Autodesk Fusion 360 part; units mm, degrees
sketch "Sketch3" plane through (0, 0, 0) normal (0, 1, 0) x (1, 0, 0)
  line L0 (42, -10) -> (120, -10)
  line L1 (135, -25) -> (135, -59)
  line L2 (120, -74) -> (42, -74)
  line L3 (10, -42) -> (10, -42)
  arc A0 (42, -10) -> (10, -42) centre (42, -42) ccw
  arc A1 (10, -42) -> (42, -74) centre (42, -42) ccw
  arc A2 (135, -25) -> (120, -10) centre (120, -25) ccw
  arc A3 (120, -74) -> (135, -59) centre (120, -59) ccw
  circle A4 centre (120, -59) radius 6.5
  circle A5 centre (120, -25) radius 6.5
  point P0 (10, -10)
  point P1 (135, -10)
  point P2 (10, -74)
  dimension "d17" = 125
  dimension "d18" = 64
  dimension "d19" = 32
  dimension "d20" = 32
  dimension "d21" = 15
  dimension "d22" = 15
  dimension "d23" = 13
  dimension "d24" = 13
extrude "Extrude3" add sketch "Sketch3" along normal blind 20
sketch "Sketch4" plane through (0, 20, 0) normal (0, 1, 0) x (-1, 0, 0)
  circle A0 centre (-120, 59) radius 6.5
  circle A1 centre (-120, 25) radius 6.5
  arc A2 (-42, 10) -> (-42, 74) centre (-42, 42) ccw
  line L0 (-42, 74) -> (-120, 74)
  arc A3 (-120, 74) -> (-135, 59) centre (-120, 59) ccw
  line L1 (-135, 59) -> (-135, 25)
  arc A4 (-135, 25) -> (-120, 10) centre (-120, 25) ccw
  line L2 (-120, 10) -> (-42, 10)
  line L3 (-120, 59) -> (-72, 59)
  line L4 (-120, 25) -> (-72, 25)
  line L5 (-72, 59) -> (-72, 25)
  line L6 (-72, 59) -> (-72, 42)
  circle A5 centre (-72, 42) radius 30
  dimension "d27" = 48
  dimension "d28" = 48
  dimension "d29" = 60
extrude "Extrude4" add sketch "Sketch4" along normal blind 45 contours L3 L4 L5 L6 A5 | L3 L4 L5 L6 A5
hole "Hole1" at (72, 65, 42) direction (0, -1, 0) diameter 30 depth 90 tip angle 118
sketch "Sketch5" plane through (0, 0, 74) normal (0, 0, 1) x (1, 0, 0)
  line L0 (42, 0) -> (120, 0)
  line L1 (120, 0) -> (120, 20)
  line L2 (120, 20) -> (42, 20)
  line L3 (42, 20) -> (42, 0)
sketch "Sketch6" plane through (0, 0, 0) normal (0, 0, 1) x (1, 0, 0)
  line L0 (42, 65) -> (72, 65)
  line L1 (42, 65) -> (42, 57.5)
  line L2 (42, 57.5) -> (57, 57.5)
  line L3 (57, 57.5) -> (87, 57.5)
  line L4 (87, 57.5) -> (87, 27.5)
  line L5 (87, 27.5) -> (57, 27.5)
  line L6 (57, 27.5) -> (57, 57.5)
  dimension "d35" = 30
  dimension "d36" = 7.5
  dimension "d37" = 30
  dimension "d38" = 30
extrude "Extrude5" cut sketch "Sketch6" along normal blind 200
sketch "Sketch7" plane through (0, 0, 0) normal (0, 1, 0) x (1, 0, 0)
sketch "Sketch8" plane through (0, 20, 0) normal (0, 1, 0) x (-1, 0, 0)
  circle A0 centre (-72, 42) radius 30
  circle A1 centre (-120, 59) radius 6.5
  circle A2 centre (-120, 25) radius 6.5
  arc A3 (-42, 10) -> (-42, 74) centre (-42, 42) ccw
  line L0 (-42, 74) -> (-120, 74)
  arc A4 (-120, 74) -> (-135, 59) centre (-120, 59) ccw
  line L1 (-135, 59) -> (-135, 25)
  arc A5 (-135, 25) -> (-120, 10) centre (-120, 25) ccw
  line L2 (-120, 10) -> (-42, 10)
  line L3 (-72, 42) -> (-27, 42)
  circle A6 centre (-27, 42) radius 6.5
  dimension "d41" = 45
  dimension "d42" = 13
extrude "Extrude6" cut sketch "Sketch8" against normal blind 9 contours A6
sketch "Sketch9" plane through (0, 20, 0) normal (0, 1, 0) x (-1, 0, 0)
  circle A0 centre (-27, 42) radius 6.5
  circle A1 centre (-72, 42) radius 30
  circle A2 centre (-120, 59) radius 6.5
  circle A3 centre (-120, 25) radius 6.5
  arc A4 (-42, 10) -> (-42, 74) centre (-42, 42) ccw
  line L0 (-42, 74) -> (-120, 74)
  arc A5 (-120, 74) -> (-135, 59) centre (-120, 59) ccw
  line L1 (-135, 59) -> (-135, 25)
  arc A6 (-135, 25) -> (-120, 10) centre (-120, 25) ccw
  line L2 (-120, 10) -> (-42, 10)
  line L3 (-27, 42) -> (-27, 31)
  line L4 (-27, 31) -> (-6.9654, 31)
  line L5 (-6.9654, 31) -> (-6.9654, 50)
  line L6 (-6.9654, 50) -> (-6.9654, 31)
  line L7 (-27, 42) -> (-27, 53)
  line L8 (-27, 53) -> (-28, 53)
  line L9 (-38, 43) -> (-38, 41)
  line L10 (-38, 31) -> (-27, 31)
  line L11 (-27, 31) -> (-27, 53)
  line L12 (-28, 31) -> (-6, 31)
  line L13 (-6, 31) -> (-6, 53)
  line L14 (-6, 53) -> (-38, 53)
  line L15 (-38, 53) -> (-38, 31)
  arc A7 (-38, 41) -> (-28, 31) centre (-28, 41) ccw
  arc A8 (-28, 53) -> (-38, 43) centre (-28, 43) ccw
  point P0 (-38, 53)
  dimension "d45" = 11
  dimension "d46" = 11
  dimension "d47" = 11
  dimension "d48" = 22
  dimension "d49" = 32
  dimension "d50" = 22
  dimension "d51" = 10
  dimension "d52" = 10
extrude "Extrude7" cut sketch "Sketch9" against normal blind 9 contours A0 A4 L3 L4 L7 L11 L12 L14 | A0 L3 L7 L8 L9 L10 L11 L12 L14 L15 A7 A8
hole "Hole2" at (27.171, 11, 42.0282) direction (0, -1, 0) diameter 12 depth 13 tip angle 118
Read the model definition and answer for the solid it produces. Units are mm, in the model's axes. A direction names the side the tool comes from. Round coordinates to 2 decimals unless told otherwise and drop trailing zeros. Loops run counter-clockwise (first coordinate to the right, second up) from the corner with the lowest first, then second, coordinate; pieces in that order, holes last. Notation, with made-up numbers: (61.5, 86.5) -> (68.5, 86.5) arc R30 cw to (68.5, 120.5) -> close; hole circle Ø6 at (40.5, 58). An arc over 180 degrees is marked (long way). One line per item, written item: value.
1) A cutting plane is placed at C-C (z = 46). Determine the outline of the cut face in (x, y).
Answer list:
outline: (10.25, 0) -> (22.67, 0) -> (22.67, 11) -> (10.25, 11) -> close; (31.67, 0) -> (57.54, 0) -> (57.54, 27.5) -> (57, 27.5) -> (57, 57.5) -> (57.54, 57.5) -> (57.54, 65) -> (42.27, 65) -> (42.27, 20) -> (37.54, 20) -> (37.54, 11) -> (31.67, 11) -> close; (86.46, 0) -> (135, 0) -> (135, 20) -> (101.73, 20) -> (101.73, 65) -> (86.46, 65) -> (86.46, 57.5) -> (87, 57.5) -> (87, 27.5) -> (86.46, 27.5) -> close
2) A cutting plane is placed at D-D (y = 9). Determine the outline of the cut face in (x, z).
Answer list:
outline: (42, 10) -> (120, 10) arc R15 ccw to (135, 25) -> (135, 59) arc R15 ccw to (120, 74) -> (42, 74) arc R32 ccw to start; hole circle Ø12 at (27.17, 42.03); hole circle Ø30 at (72, 42); hole circle Ø13 at (120, 25); hole circle Ø13 at (120, 59)
3) A cutting plane is placed at B-B (z = 64). Determine the outline of the cut face in (x, y).
Answer list:
outline: (18.76, 0) -> (115.85, 0) -> (115.85, 20) -> (92.4, 20) -> (92.4, 65) -> (51.6, 65) -> (51.6, 20) -> (18.76, 20) -> close; (124.15, 0) -> (134.14, 0) -> (134.14, 20) -> (124.15, 20) -> close; hole (57, 27.5) -> (87, 27.5) -> (87, 57.5) -> (57, 57.5) -> close
4) The mould has two halves that part along Y. Classify faces 4 (the face through (72, 57.5, 63)), 5 (the face through (100, 20, 56)), 6 (the face through (34.99, 15.56, 50.15)): pulls with the +Y half, pulls with the -Y half, needs draft (parallel to the pull), parting line crosses it, or undercut.
Answer list:
face 4: undercut
face 5: pulls with the +Y half
face 6: needs draft
5) For faces 1 (the face through (114.842, 9.86, 55.045)), 2 (the face through (20, 16, 31)), 3 (the face through (87, 43, 42)), determine the directions among +Z, -Z, +X, -X, +Y, -Y from which every point of the face is accessible in a straight line to the end or side of a thin tool.
Answer list:
face 1: +Y, -Y
face 2: -X, +Y
face 3: +Z, -Z
6) Consider L1, parallel to Z at x = 120, y = 5; L2, parallel to X at y = 60, z = 42; L3, parallel to Z at x = 72, y = 61.25. Determine where each line is inside the solid, lowest interval first. Write a range as [from, to].
Answer list:
L1: z = [10, 18.5], [31.5, 52.5], [65.5, 74]
L2: x = [42, 57], [87, 102]
L3: z = [12, 27], [57, 72]
7) A cutting plane is placed at A-A (x = 72). Determine the outline of the cut face in (y, z), and give its area (3 significant figures).
Answer list:
outline: (0, 10) -> (20, 10) -> (20, 12) -> (27.5, 12) -> (27.5, 27) -> (0, 27) -> close; (0, 57) -> (27.5, 57) -> (27.5, 72) -> (20, 72) -> (20, 74) -> (0, 74) -> close; (57.5, 12) -> (65, 12) -> (65, 27) -> (57.5, 27) -> close; (57.5, 57) -> (65, 57) -> (65, 72) -> (57.5, 72) -> close
area: 1,130 mm²
8) Flat-ended cylindrical pins translate along their axes: P1, Ø1.5, axis at x = 46, y = 38, coming from the +Z side; P2, Ø24, axis at y = 42, z = 46, coming from the +X side; P3, Ø10, axis at y = 23, z = 29.5, coming from the -X side. Find the tip coordinate at first contact, or state that the pin passes through.
Answer list:
P1: stops at z = 58.2
P2: stops at x = 102
P3: stops at x = 11.95
